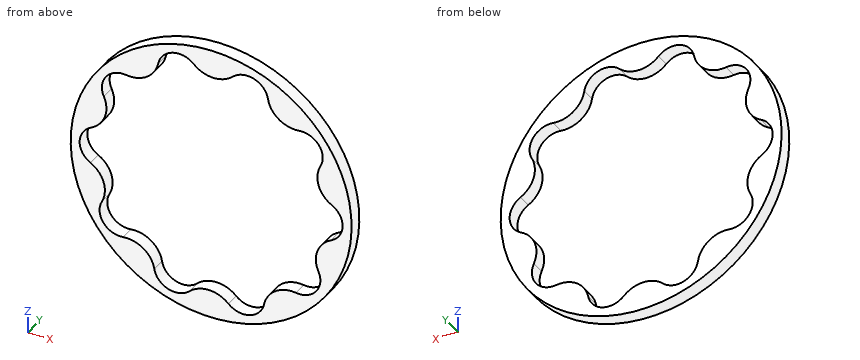
```python
from build123d import *

# Parameters (mm, degrees)
SKETCH1_R           = 100
BOSS_EXTRUDE1_DEPTH = 10


with BuildPart() as part:
    # Sketch1 → Boss-Extrude1 (new body)
    with BuildSketch(Plane(origin=(0, 0, 0), x_dir=(1, 0, 0), z_dir=(0, 1, 0))):
        with Locations(Location((0, 0, 0), (0, 0, 270))):
            Circle(SKETCH1_R)
        with BuildLine():
            ThreePointArc((-40.455763136, 76.710865294), (-30.532781322, 88.532885217), (-15.431871826, 85.340980525))
            ThreePointArc((-15.431871826, 85.340980525), (-1.435318351, 79.986408862), (12.360115413, 85.839694617))
            ThreePointArc((12.360115413, 85.839694617), (27.336785299, 89.571327274), (37.677523206, 78.112930236))
            ThreePointArc((37.677523206, 78.112930236), (45.853634574, 65.554023048), (60.454849979, 62.180678181))
            ThreePointArc((60.454849979, 62.180678181), (74.764629078, 56.396566729), (76.395384986, 41.048395558))
            ThreePointArc((76.395384986, 41.048395558), (75.6280576, 26.082228528), (85.457886638, 14.770756123))
            ThreePointArc((85.457886638, 14.770756123), (93.634925706, 1.680234544), (85.932806285, -11.69523104))
            ThreePointArc((85.932806285, -11.69523104), (76.515133126, -23.352090786), (77.818915207, -38.281092734))
            ThreePointArc((77.818915207, -38.281092734), (76.739863248, -53.677890129), (62.646816331, -59.971676886))
            ThreePointArc((62.646816331, -59.971676886), (48.176028451, -63.866705129), (40.455763136, -76.710865294))
            ThreePointArc((40.455763136, -76.710865294), (30.532781322, -88.532885217), (15.431871826, -85.340980525))
            ThreePointArc((15.431871826, -85.340980525), (1.435318351, -79.986408862), (-12.360115413, -85.839694617))
            ThreePointArc((-12.360115413, -85.839694617), (-27.336785299, -89.571327274), (-37.677523206, -78.112930236))
            ThreePointArc((-37.677523206, -78.112930236), (-45.853634574, -65.554023048), (-60.454849979, -62.180678181))
            ThreePointArc((-60.454849979, -62.180678181), (-74.764629078, -56.396566729), (-76.395384986, -41.048395558))
            ThreePointArc((-76.395384986, -41.048395558), (-75.6280576, -26.082228528), (-85.457886638, -14.770756123))
            ThreePointArc((-85.457886638, -14.770756123), (-93.634925706, -1.680234544), (-85.932806285, 11.69523104))
            ThreePointArc((-85.932806285, 11.69523104), (-76.515133126, 23.352090786), (-77.818915207, 38.281092734))
            ThreePointArc((-77.818915207, 38.281092734), (-76.739863248, 53.677890129), (-62.646816331, 59.971676886))
            ThreePointArc((-62.646816331, 59.971676886), (-48.176028451, 63.866705129), (-40.455763136, 76.710865294))
        make_face(mode=Mode.SUBTRACT)
    extrude(amount=BOSS_EXTRUDE1_DEPTH)


solid = part.part
```
The model under review builds one solid part; all positions refer to its coordinate system, in mm. Give positions to 0.01 mm unless a question says otherwise; leave off trailing zeros. Loops run counter-clockwise (first coordinate to the right, second up) from the corner with the lowest first, then second, coordinate; pieces in that order, holes last. Notation, with made-up numbers: (-38.75, 80.25) - (-30.75, 80.25) arc R26 ccw to (-30.75, 111.25) - close; hole circle Ø3 at (27, 26.25). An arc over 180 degrees is marked (long way). Answer as a JSON object with one key per item and string values.
Q1. Insertion check: pin 1 (1.5 mm diameter, centred on y = 2.5, z = -19, fed in from +X); pin 2 (1 mm diameter, centred on x = 39, y = 4.5, fed in from -Z); pin 3 (5 mm diameter, centred on y = 6, z = -58.5, fed in from +X). Each pin has a flat end and moves straight along its axis. Give the tip position at first contact, or say it passes through.
Worked out:
{"pin 1": "stops at x = 98.32", "pin 2": "stops at z = -92.29", "pin 3": "stops at x = 82.85"}
Q2. Add section A-A on x = -83. State the section outline as (y, z) points, plus the area to 3 significant figures.
Worked out:
{"outline": "(0, -55.78) - (10, -55.78) - (10, -13.69) - (0, -13.69) - close; (0, 16.26) - (10, 16.26) - (10, 55.78) - (0, 55.78) - close", "area": "816 mm^2"}
Q3. To check wall thickness, follow line 1 along Z through (x, y) = (55, 6); line 2 along Z through (x, y) = (6.5, 3); line 3 along X through (y, z) = (1.5, -25.5). State the ranges of each line that lie inside material, in increasing order.
Worked out:
{"line 1": "z = -83.52 to -62.07, 60.52 to 83.52", "line 2": "z = -99.79 to -81.78, 80.54 to 99.79", "line 3": "x = -96.69 to -75.99, 75.84 to 96.69"}
Q4. Add section B-B on z = 0. State the section outline as (x, y) points, plus the area to 3 significant figures.
Worked out:
{"outline": "(-100, 0) - (-93.57, 0) - (-93.57, 10) - (-100, 10) - close; (93.57, 0) - (100, 0) - (100, 10) - (93.57, 10) - close", "area": "129 mm^2"}
Q5. Add section C-C on y = 7.75. State the section outline as (x, z) points, plus the area to 3 significant figures.
Worked out:
{"outline": "circle Ø200 at (0, 0); hole (-85.93, -11.7) arc R20.03 cw to (-77.82, -38.28) arc R15 ccw to (-62.65, -59.97) arc R20.03 cw to (-40.46, -76.71) arc R15 ccw to (-15.43, -85.34) arc R20.03 cw to (12.36, -85.84) arc R15 ccw to (37.68, -78.11) arc R20.03 cw to (60.45, -62.18) arc R15 ccw to (76.4, -41.05) arc R20.03 cw to (85.46, -14.77) arc R15 ccw to (85.93, 11.7) arc R20.03 cw to (77.82, 38.28) arc R15 ccw to (62.65, 59.97) arc R20.03 cw to (40.46, 76.71) arc R15 ccw to (15.43, 85.34) arc R20.03 cw to (-12.36, 85.84) arc R15 ccw to (-37.68, 78.11) arc R20.03 cw to (-60.45, 62.18) arc R15 ccw to (-76.4, 41.05) arc R20.03 cw to (-85.46, 14.77) arc R15 ccw to start", "area": "7,750 mm^2"}
